The listing builds one solid part. Answer for the finished solid, in the listing's coordinates (mm). A direction names the side the tool comes from. Coordinates: 2 decimals unless noted, no trailing zeros. Loops run counter-clockwise (first coordinate to the right, second up) from the corner with the lowest first, then second, coordinate; pieces in that order, holes last. Notation, with made-up numbers: (27, 38.5) - (61, 38.5) arc R14 cw to (61, 60.5) - close; hole circle Ø8 at (80.25, -25). An arc over 180 degrees is marked (long way). Return JSON: item names as keys, results as strings. Group by question number.
1. Section B-B (x = 0) is taken. Write down the section's boundary in (y, z).
2. Which of the six approach directions +Z, -Z, +X, -X, +Y, -Y give full straight-line access (tool end or side, diameter ignored) to faces 4 (the face through (4, 2, 16)), 5 (the face through (-4, 3, 8)), 6 (the face through (1, 5.5, 13)), 7 (the face through (-4, 3.5, 16))?
3. Each of these flat-tipped pins is pushed along its axis until it touches: P1, Ø1.6, axis at x = 3.5, z = 12, coming from the +Y side; P2, Ø1, axis at x = -4, z = 13, coming from the -Y side; P3, Ø1.6, axis at x = 4, y = 3, coming from the -Z side; P4, Ø1.6, axis at x = -3.5, y = 17.5, coming from the -Z side. Where does it stop, or does it pass through?
4. Find the intervals of material crossed by line 1 along Z through (x, y) = (0, 1.25); line 2 along X through (y, z) = (3.4, 15); line 3 along X through (y, z) = (2.5, 7.5), in increasing order.
5. Section A-A (z = 15) is taken. Write down the section's boundary in (x, y), and give its area (3 significant figures).
6. The mould has two halves that part along X. Classify faces 1 (the face through (-5, 16, 3)), 2 (the face through (4, 3.5, 16)), 3 (the face through (0.487, 2.783, 16.546)): pulls with the +X half, pulls with the -X half, needs draft (parallel to the pull), parting line crosses it, or undercut.
7. Section D-D (x = -4.25) is taken. Write down the section's boundary in (y, z).
Autodesk Inventor part; units mm, degrees
ref_plane "bracket_to_screw1_XY" through (0, 15, 5) normal (0, 0, -1) x (1, 0, 0)
ref_plane "bracket_to_screw1_YZ" through (0, 15, 5) normal (1, 0, 0) x (0, -1, 0)
ref_plane "bracket_to_screw1_ZX" through (0, 15, 5) normal (0, -1, 0) x (0, 0, -1)
sketch "Sketch_12" plane through (0, 0, 0) normal (0, 0, 1) x (1, 0, 0)
  line L0 (-2.95, 0) -> (2.95, 0)
  line L1 (2.95, 0) -> (2.95, 5.5)
  line L2 (2.95, 5.5) -> (-2.95, 5.5)
  line L3 (-2.95, 5.5) -> (-2.95, 0)
extrude "Extrusion1" add sketch "Sketch_12" along normal blind 23
sketch "Sketch_9" plane through (0, 0, 23) normal (0, 0, 1) x (1, 0, 0)
  line L0 (-5, 2) -> (5, 2)
  line L1 (5, 2) -> (5, 3.5)
  line L2 (5, 3.5) -> (-5, 3.5)
  line L3 (-5, 3.5) -> (-5, 2)
extrude "Extrusion2" add sketch "Sketch_9" against normal blind 15
sketch "Sketch_8" plane through (0, 0, 0) normal (0, 1, 0) x (-1, 0, 0)
  line L0 (2.95, 5.5) -> (-2.95, 5.5)
  line L1 (-2.95, 5.5) -> (-2.95, 0)
  line L2 (-2.95, 0) -> (2.95, 0)
  line L3 (2.95, 0) -> (2.95, 5.5)
extrude "Extrusion3" add sketch "Sketch_8" along normal blind 23
sketch "Sketch_2" plane through (0, 23, 0) normal (0, 1, 0) x (1, 0, 0)
  line L0 (-5, -3.5) -> (5, -3.5)
  line L1 (5, -3.5) -> (5, -2)
  line L2 (5, -2) -> (-5, -2)
  line L3 (-5, -2) -> (-5, -3.5)
extrude "Extrusion4" add sketch "Sketch_2" against normal blind 15
sketch "Sketch_4" plane through (0, 0, 0) normal (1, 0, 0) x (0, 1, 0)
  line L0 (5.5, 15) -> (0, 15)
  line L1 (0, 15) -> (0, 17)
  line L2 (0, 17) -> (0.379, 16.621)
  line L3 (0.379, 16.621) -> (5.121, 16.621)
  line L4 (5.121, 16.621) -> (5.5, 17)
  line L5 (5.5, 17) -> (5.5, 15)
  line L6 (5.5, 15) -> (0, 15)
revolve "Revolution1" cut sketch "Sketch_4" angle 360 about axis through (0, 5.5, 15) along (0, -1, 0)
thread "Thread1"
sketch "Sketch_5" plane through (0, 0, 0) normal (1, 0, 0) x (0, 1, 0)
  line L0 (15, 0) -> (15, 5.5)
  line L1 (15, 5.5) -> (17, 5.5)
  line L2 (17, 5.5) -> (16.621, 5.121)
  line L3 (16.621, 5.121) -> (16.621, 0.379)
  line L4 (16.621, 0.379) -> (17, 0)
  line L5 (17, 0) -> (15, 0)
  line L6 (15, 0) -> (15, 5.5)
revolve "Revolution2" cut sketch "Sketch_5" angle 360 about axis through (0, 15, 0) along (0, 0, 1)
thread "Thread2"
sketch "_____1" plane through (0, 0, 0) normal (1, 0, 0) x (0, 0, -1)
  line L0 (-7.1, 5.5) -> (-5.5, 5.5)
  line L1 (-5.5, 5.5) -> (-5.5, 7.1)
  arc A0 (-7.1, 5.5) -> (-5.5, 7.1) centre (-7.1, 7.1) ccw
extrude "Extrusion5" add sketch "_____1" along normal mid plane 5.9
sketch "_____2" plane through (0, 0, 0) normal (1, 0, 0) x (0, 0, -1)
  line L0 (-1, 0) -> (0, 0)
  line L1 (0, 0) -> (0, 1)
  arc A0 (-1, 0) -> (0, 1) centre (-1, 1) ccw
extrude "Extrusion6" cut sketch "_____2" along normal mid plane 5.9
ref_plane "bracket_to_screw1_XY" through (0, 15, 5) normal (0, 0, -1) x (1, 0, 0)
ref_plane "bracket_to_screw1_YZ" through (0, 15, 5) normal (1, 0, 0) x (0, -1, 0)
ref_plane "bracket_to_screw1_ZX" through (0, 15, 5) normal (0, -1, 0) x (0, 0, -1)
ref_plane "bracket_to_screw2_XY" through (0, 5, 15) normal (0, -1, 0) x (1, 0, 0)
ref_plane "bracket_to_screw2_YZ" through (0, 5, 15) normal (1, 0, 0) x (0, 0, 1)
ref_plane "bracket_to_screw2_ZX" through (0, 5, 15) normal (0, 0, 1) x (0, -1, 0)
properties part number "HBLBS5b"
The answers:
{
 "1": {"outline": "(0, 1) arc R1 ccw to (1, 0) - (13, 0) - (13.38, 0.38) - (13.38, 5.12) - (13, 5.5) - (7.1, 5.5) arc R1.6 cw to (5.5, 7.1) - (5.5, 13) - (5.12, 13.38) - (0.38, 13.38) - (0, 13) - close; (0, 17) - (0.38, 16.62) - (5.12, 16.62) - (5.5, 17) - (5.5, 23) - (0, 23) - close; (16.62, 0.38) - (17, 0) - (23, 0) - (23, 5.5) - (17, 5.5) - (16.62, 5.12) - close"},
 "2": {"face 4": "+Z, -Z, +X, -Y", "face 5": "-Z, -X, +Y, -Y", "face 6": "+Z, +X, -X, +Y", "face 7": "+Z, -Z, -X, +Y"},
 "3": {"P1": "stops at y = 5.5", "P2": "stops at y = 2", "P3": "stops at z = 8", "P4": "stops at z = 0"},
 "4": {"line 1": "z = 0 to 13.38, 16.62 to 23", "line 2": "x = -5 to -1.62, 1.62 to 5", "line 3": "x = -2.95 to 2.95"},
 "5": {"outline": "(-5, 2) - (-2.95, 2) - (-2.95, 0) - (-2, 0) - (-1.62, 0.38) - (-1.62, 5.12) - (-2, 5.5) - (-2.95, 5.5) - (-2.95, 3.5) - (-5, 3.5) - close; (1.62, 0.38) - (2, 0) - (2.95, 0) - (2.95, 2) - (5, 2) - (5, 3.5) - (2.95, 3.5) - (2.95, 5.5) - (2, 5.5) - (1.62, 5.12) - close", "area": "20.5 mm2"},
 "6": {"face 1": "pulls with the -X half", "face 2": "needs draft", "face 3": "undercut"},
 "7": {"outline": "(2, 8) - (3.5, 8) - (3.5, 23) - (2, 23) - close; (8, 2) - (23, 2) - (23, 3.5) - (8, 3.5) - close"}
}
